```python
from build123d import *

# Parameters (mm, degrees)
F1_DEPTH = 25.4
F3_DEPTH = 1.27
F4_DEPTH = 1.27


with BuildPart() as f1:
    # F0 (on Right) → F1 (new body)
    with BuildSketch(Plane.YZ):
        with BuildLine():
            ThreePointArc((5.4992613166, -3.1749999956), (6.1336289976, -1.6435009339), (6.35, 0))
            ThreePointArc((6.35, 0), (6.1336289982, 1.6435009317), (5.4992613189, 3.1749999916))
            ThreePointArc((5.4992613189, 3.1749999916), (3.1750000042, 5.4992613116), (0, 6.35))
            ThreePointArc((0, 6.35), (-3.1750000022, 5.4992613128), (-5.4992613166, 3.1749999956))
            ThreePointArc((-5.4992613166, 3.1749999956), (-6.35, 5.57e-08), (-5.4992613723, -3.1749998991))
            ThreePointArc((-5.4992613723, -3.1749998991), (-3.1750000504, -5.4992612849), (0, -6.35))
            ThreePointArc((0, -6.35), (3.1750000022, -5.4992613128), (5.4992613166, -3.1749999956))
        make_face()
    extrude(amount=F1_DEPTH)

    # F2 (on face) → F3 (join)
    with BuildSketch(Plane.YZ.offset(25.4)):
        with BuildLine():
            ThreePointArc((3.1750003445, -5.4992611151), (5.4992614135, -3.1749998278), (6.35, 0))
            ThreePointArc((6.35, 0), (5.4992613234, 3.1749999838), (3.1750000324, 5.4992612953))
            ThreePointArc((3.1750000324, 5.4992612953), (5.57e-08, 6.35), (-3.174999936, 5.499261351))
            ThreePointArc((-3.174999936, 5.499261351), (-5.4992612955, 3.175000032), (-6.35, 0))
            ThreePointArc((-6.35, 0), (-5.4992613963, -3.1749998576), (-3.1750002849, -5.4992611496))
            ThreePointArc((-3.1750002849, -5.4992611496), (3.44e-08, -6.35), (3.1750003445, -5.4992611151))
        make_face()
        with BuildLine():
            Line((6.35, 0), (6.35, 3.6661742094))
            Line((6.35, 3.6661742094), (3.1750000324, 5.4992612953))
            ThreePointArc((3.1750000324, 5.4992612953), (5.4992613234, 3.1749999838), (6.35, 0))
        make_face()
        with BuildLine():
            Line((-6.35, -3.6661742094), (-3.1750002849, -5.4992611496))
            ThreePointArc((-3.1750002849, -5.4992611496), (-5.4992613963, -3.1749998576), (-6.35, 0))
            Line((-6.35, 0), (-6.35, -3.6661742094))
        make_face()
        with BuildLine():
            Line((6.35, -3.6661742094), (6.35, 0))
            ThreePointArc((6.35, 0), (5.4992614135, -3.1749998278), (3.1750003445, -5.4992611151))
            Line((3.1750003445, -5.4992611151), (6.35, -3.6661742094))
        make_face()
        with BuildLine():
            ThreePointArc((-3.174999936, 5.499261351), (5.57e-08, 6.35), (3.1750000324, 5.4992612953))
            Line((3.1750000324, 5.4992612953), (0, 7.3323484187))
            Line((0, 7.3323484187), (-3.174999936, 5.499261351))
        make_face()
        with BuildLine():
            Line((0, -7.3323484187), (3.1750003445, -5.4992611151))
            ThreePointArc((3.1750003445, -5.4992611151), (3.44e-08, -6.35), (-3.1750002849, -5.4992611496))
            Line((-3.1750002849, -5.4992611496), (0, -7.3323484187))
        make_face()
        with BuildLine():
            ThreePointArc((-6.35, 0), (-5.4992612955, 3.175000032), (-3.174999936, 5.499261351))
            Line((-3.174999936, 5.499261351), (-6.35, 3.6661742094))
            Line((-6.35, 3.6661742094), (-6.35, 0))
        make_face()
    extrude(amount=F3_DEPTH)

    # F0 (on Right) → F4 (join)
    with BuildSketch(Plane.YZ):
        with BuildLine():
            ThreePointArc((5.4992613189, 3.1749999916), (6.1336289982, 1.6435009317), (6.35, 0))
            ThreePointArc((6.35, 0), (6.1336289976, -1.6435009339), (5.4992613166, -3.1749999956))
            Line((5.4992613166, -3.1749999956), (7.3323484187, 0))
            Line((7.3323484187, 0), (5.4992613189, 3.1749999916))
        make_face()
        with BuildLine():
            ThreePointArc((-5.4992613723, -3.1749998991), (-6.35, 5.57e-08), (-5.4992613166, 3.1749999956))
            Line((-5.4992613166, 3.1749999956), (-7.3323484187, 0))
            Line((-7.3323484187, 0), (-5.4992613723, -3.1749998991))
        make_face()
        with BuildLine():
            ThreePointArc((0, 6.35), (3.1750000042, 5.4992613116), (5.4992613189, 3.1749999916))
            Line((5.4992613189, 3.1749999916), (3.6661742094, 6.35))
            Line((3.6661742094, 6.35), (0, 6.35))
        make_face()
        with BuildLine():
            Line((3.6661742094, -6.35), (5.4992613166, -3.1749999956))
            ThreePointArc((5.4992613166, -3.1749999956), (3.1750000022, -5.4992613128), (0, -6.35))
            Line((0, -6.35), (3.6661742094, -6.35))
        make_face()
        with BuildLine():
            ThreePointArc((-5.4992613166, 3.1749999956), (-3.1750000022, 5.4992613128), (0, 6.35))
            Line((0, 6.35), (-3.6661742094, 6.35))
            Line((-3.6661742094, 6.35), (-5.4992613166, 3.1749999956))
        make_face()
        with BuildLine():
            Line((-3.6661742094, -6.35), (0, -6.35))
            ThreePointArc((0, -6.35), (-3.1750000504, -5.4992612849), (-5.4992613723, -3.1749998991))
            Line((-5.4992613723, -3.1749998991), (-3.6661742094, -6.35))
        make_face()
        with BuildLine():
            ThreePointArc((5.4992613166, -3.1749999956), (6.1336289976, -1.6435009339), (6.35, 0))
            ThreePointArc((6.35, 0), (6.1336289982, 1.6435009317), (5.4992613189, 3.1749999916))
            ThreePointArc((5.4992613189, 3.1749999916), (3.1750000042, 5.4992613116), (0, 6.35))
            ThreePointArc((0, 6.35), (-3.1750000022, 5.4992613128), (-5.4992613166, 3.1749999956))
            ThreePointArc((-5.4992613166, 3.1749999956), (-6.35, 5.57e-08), (-5.4992613723, -3.1749998991))
            ThreePointArc((-5.4992613723, -3.1749998991), (-3.1750000504, -5.4992612849), (0, -6.35))
            ThreePointArc((0, -6.35), (3.1750000022, -5.4992613128), (5.4992613166, -3.1749999956))
        make_face()
    extrude(amount=-F4_DEPTH)


solid = f1.part
```
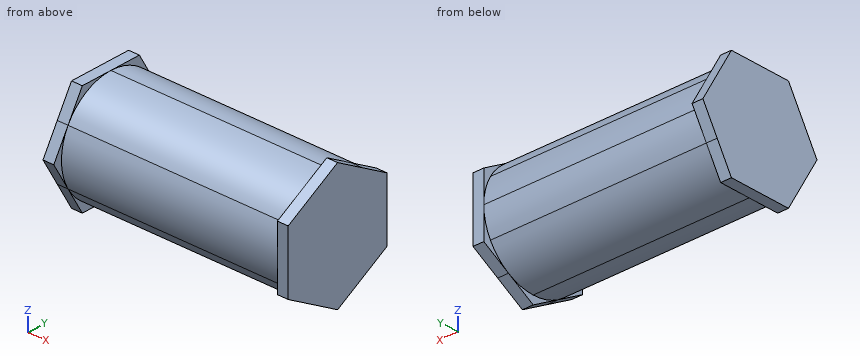
Input: part model. Units: mm. Frame: model coordinates. Coordinates: 2 decimals unless noted, no trailing zeros. Loops run counter-clockwise (first coordinate to the right, second up) from the corner with the lowest first, then second, coordinate; pieces in that order, holes last. Notation, with made-up numbers: M 76,43 L 96,43 A28 ccw 96,73 Z; hole C 55.5,-22.5 d11. An arc over 180 degrees is marked long. Answer in a Markdown table with one row per item.
1. Material intervals for line 1 (Y direction, x = 21.75, z = 0.25); line 2 (Z direction, x = 10, y = 4.5); line 3 (Z direction, x = 3, y = 2), sorted ascending.
Response:
| item | result |
|---|---|
| line 1 | y = -6.35 to 6.35 |
| line 2 | z = -4.48 to 4.48 |
| line 3 | z = -6.03 to 6.03 |
2. First-contact query: pin 1 (2 mm diameter, centred on x = 14.5, z = 3.5, fed in from -Y); pin 2 (3 mm diameter, centred on x = 2, y = 3, fed in from +Z); pin 3 (3 mm diameter, centred on x = 6, y = 3.5, fed in from -Z). Flat tips, straight axial feed; report the tip coordinate or a pass-through.
Response:
| item | result |
|---|---|
| pin 1 | stops at y = -5.84 |
| pin 2 | stops at z = 6.17 |
| pin 3 | stops at z = -6.03 |
3. Section B-B, the plane z = -5. Output: boundary loops of the cut face in (x, y).
Response:
| item | result |
|---|---|
| outline | M -1.27,-4.45 L 0,-4.45 L 0,-3.91 L 25.4,-3.91 L 25.4,-4.04 L 26.67,-4.04 L 26.67,4.04 L 25.4,4.04 L 25.4,3.91 L 0,3.91 L 0,4.45 L -1.27,4.45 Z |
4. Section A-A, the plane x = 11. Output: boundary loops of the cut face in (y, z) (3 decimals).
Response:
| item | result |
|---|---|
| outline | C 0,0 d12.7 |
